```python
from build123d import *

# Parameters (mm, degrees)
F0_W     = 362.293
F0_H     = 210
F1_DEPTH = 135
F2_R     = 40
F3_DEPTH = 40
F5_DEPTH = 210.001
F6_R     = 37.5
F7_DEPTH = 362.294


with BuildPart() as f1:
    # F0 (on Front) → F1 (new body)
    with BuildSketch(Plane.XZ):
        Rectangle(F0_W, F0_H)
    extrude(amount=-F1_DEPTH)

    # F2 (on face) → F3 (join)
    with BuildSketch(Plane(origin=(0, 135, 0), x_dir=(-1, 0, 0), z_dir=(0, 1, 0))):
        Circle(F2_R)
    extrude(amount=F3_DEPTH)

    # F4 (on face) → F5 (cut, through all)
    with BuildSketch(Plane(origin=(0, 0, -105), x_dir=(1, 0, 0), z_dir=(0, 0, -1))):
        Polygon((0, 0), (-33.8, 0), (-33.8, -90), (33.8, -90), (33.8, 0), align=None)
    extrude(amount=-F5_DEPTH, mode=Mode.SUBTRACT)

    # F6 (on face) → F7 (cut, through all)
    with BuildSketch(Plane(origin=(-181.1465, 0, 0), x_dir=(0, -1, 0), z_dir=(-1, 0, 0))):
        with Locations((-50, 50)):
            Circle(F6_R)
        with Locations((-50, -50)):
            Circle(F6_R)
    extrude(amount=-F7_DEPTH, mode=Mode.SUBTRACT)


solid = f1.part
```
Work out the finished part from the listing and answer in its coordinate system (mm). A direction names the side the tool comes from. Coordinates: 2 decimals unless noted, no trailing zeros. Loops run counter-clockwise (first coordinate to the right, second up) from the corner with the lowest first, then second, coordinate; pieces in that order, holes last.
1) Section C-C (x = 0) is taken. Give the vertices of the cut face in (y, z).
Results:
outline: (90, -105) - (135, -105) - (135, -40) - (175, -40) - (175, 40) - (135, 40) - (135, 105) - (90, 105) - close
2) For faces 1 (the cylindrical face through (-108.5, 15.36, -64.36)), 2 (the cylindrical face through (8.67, 154.72, -39.05)), 3 (the flat face through (0, 90, -1)), determine the directions among +Z, -Z, +X, -X, +Y, -Y from which every point of the face is accessible in a straight line to the end or side of a thin tool.
Results:
face 1: +X, -X
face 2: +Y
face 3: +Z, -Z, -Y
3) Section A-A (y = 50) is taken. Give the vertices of the cut face in (x, z), plus the area to 3 significant figures.
Results:
outline: (-181.15, -105) - (-33.8, -105) - (-33.8, -87.5) - (-181.15, -87.5) - close; (-181.15, -12.5) - (-33.8, -12.5) - (-33.8, 12.5) - (-181.15, 12.5) - close; (-181.15, 87.5) - (-33.8, 87.5) - (-33.8, 105) - (-181.15, 105) - close; (33.8, -105) - (181.15, -105) - (181.15, -87.5) - (33.8, -87.5) - close; (33.8, -12.5) - (181.15, -12.5) - (181.15, 12.5) - (33.8, 12.5) - close; (33.8, 87.5) - (181.15, 87.5) - (181.15, 105) - (33.8, 105) - close
area: 17,700 mm2
4) Section D-D (x = -83) is taken. Give the vertices of the cut face in (y, z).
Results:
outline: (0, -105) - (135, -105) - (135, 105) - (0, 105) - close; hole circle Ø75 at (50, -50); hole circle Ø75 at (50, 50)
5) Flat-ended cylindrical pins translate along their axes: pin 1 (3 mm diameter, centred on x = -31, z = -63, fed in from -Y); pin 2 (2 mm diameter, centred on y = 140.5, z = -26, fed in from +X) (3 decimals). Find the tip coordinate at first contact, or state that the pin passes through.
Results:
pin 1: stops at y = 90
pin 2: stops at x = 31.225
6) For a pull along Y with two mould halves and no side action, classify faces 4 (the flat face through (-33.8, 34, -1)), 5 (the cylindrical face through (106.44, 32.7, 16.73)), 6 (the flat face through (1, 175, 1)) as +Y half, -Y half, draft (parallel to the pull), parting line (faces both ways), or undercut.
Results:
face 4: draft
face 5: undercut
face 6: +Y half
7) Section B-B (z = -50) is taken. Give the vertices of the cut face in (x, y), plus the area to 3 significant figures.
Results:
outline: (-181.15, 0) - (-33.8, 0) - (-33.8, 12.5) - (-181.15, 12.5) - close; (-181.15, 87.5) - (-33.8, 87.5) - (-33.8, 90) - (33.8, 90) - (33.8, 87.5) - (181.15, 87.5) - (181.15, 135) - (-181.15, 135) - close; (33.8, 0) - (181.15, 0) - (181.15, 12.5) - (33.8, 12.5) - close
area: 20,700 mm2
8) Consider probe 1 along Z at (x, y) = (99, 50); probe 2 along X at (y, z) = (85, -84.5); probe 3 along Z at (x, y) = (-131.5, 58). Determine where each line is inside the solid, lowest interval first.
Results:
probe 1: z = -105 to -87.5, -12.5 to 12.5, 87.5 to 105
probe 2: x = -181.15 to -33.8, 33.8 to 181.15
probe 3: z = -105 to -86.64, -13.36 to 13.36, 86.64 to 105
